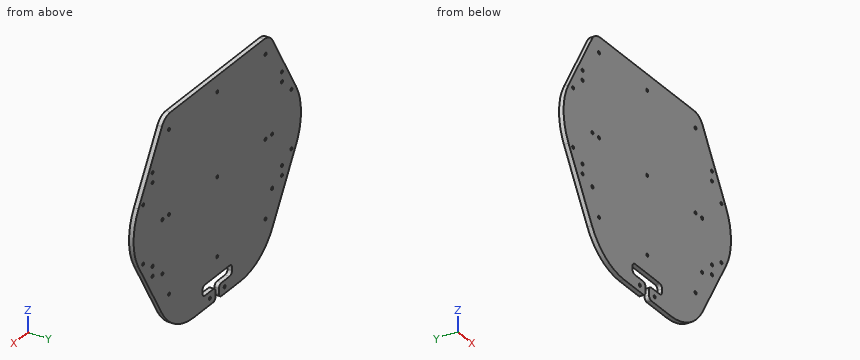
from build123d import *

# Parameters (mm, degrees)
ESBO_O1_R                = 2
ESBO_O1_R_2              = 2.1
RESSALTO_EXTRUS_O1_DEPTH = 6


with BuildPart() as part:
    # Esboço1 → Ressalto-extrusão1 (new body)
    with BuildSketch(Plane(origin=(0, 6, 0), x_dir=(1, 0, 0), z_dir=(0, 1, 0))):
        with BuildLine():
            Line((-94.999273038, -130), (94.999273038, -130))
            ThreePointArc((94.999273038, -130), (104.95780768, -127.344382024), (112.27173596, -120.082758778))
            ThreePointArc((112.27173596, -120.082758778), (112.362006236, -119.927693826), (112.451905284, -119.77241336))
            Line((112.451905284, -119.77241336), (159.951905284, -37.5))
            ThreePointArc((159.951905284, -37.5), (170, 0), (159.951905284, 37.5))
            Line((159.951905284, 37.5), (112.451905284, 119.77241336))
            ThreePointArc((112.451905284, 119.77241336), (85, 147.224318643), (47.5, 157.27241336))
            Line((47.5, 157.27241336), (8.5, 157.27241336))
            ThreePointArc((8.5, 157.27241336), (4.964466094, 155.807947265), (3.5, 152.27241336))
            Line((3.5, 152.27241336), (3.5, 145.27241336))
            ThreePointArc((3.5, 145.27241336), (4.964466094, 141.736879454), (8.5, 140.27241336))
            Line((8.5, 140.27241336), (25, 140.27241336))
            ThreePointArc((25, 140.27241336), (28.535533906, 138.807947265), (30, 135.27241336))
            Line((30, 135.27241336), (30, 131.27241336))
            ThreePointArc((30, 131.27241336), (28.535533906, 127.736879454), (25, 126.27241336))
            Line((25, 126.27241336), (-25, 126.27241336))
            ThreePointArc((-25, 126.27241336), (-28.535533906, 127.736879454), (-30, 131.27241336))
            Line((-30, 131.27241336), (-30, 135.27241336))
            ThreePointArc((-30, 135.27241336), (-28.535533906, 138.807947265), (-25, 140.27241336))
            Line((-25, 140.27241336), (-8.5, 140.27241336))
            ThreePointArc((-8.5, 140.27241336), (-4.964466094, 141.736879454), (-3.5, 145.27241336))
            Line((-3.5, 145.27241336), (-3.5, 152.27241336))
            ThreePointArc((-3.5, 152.27241336), (-4.964466094, 155.807947265), (-8.5, 157.27241336))
            Line((-8.5, 157.27241336), (-47.5, 157.27241336))
            ThreePointArc((-47.5, 157.27241336), (-85, 147.224318643), (-112.451905284, 119.77241336))
            Line((-112.451905284, 119.77241336), (-159.951905284, 37.5))
            ThreePointArc((-159.951905284, 37.5), (-170, 0), (-159.951905284, -37.5))
            Line((-159.951905284, -37.5), (-112.451905284, -119.77241336))
            ThreePointArc((-112.451905284, -119.77241336), (-112.362006236, -119.927693826), (-112.27173596, -120.082758778))
            ThreePointArc((-112.27173596, -120.082758778), (-104.95780768, -127.344382024), (-94.999273038, -130))
        make_face()
        with Locations(Location((150.5, -38.1, 0), (0, 0, 90))):
            Circle(ESBO_O1_R, mode=Mode.SUBTRACT)
        with Locations(Location((150.5, 38.1, 0), (0, 0, 90))):
            Circle(ESBO_O1_R, mode=Mode.SUBTRACT)
        with Locations(Location((-150.5, -38.1, 0), (0, 0, 90))):
            Circle(ESBO_O1_R, mode=Mode.SUBTRACT)
        with Locations(Location((-150.5, 38.1, 0), (0, 0, 90))):
            Circle(ESBO_O1_R, mode=Mode.SUBTRACT)
        with Locations(Location((15, 148.77, 0), (0, 0, 90))):
            Circle(ESBO_O1_R, mode=Mode.SUBTRACT)
        with Locations(Location((-15, 148.77, 0), (0, 0, 90))):
            Circle(ESBO_O1_R, mode=Mode.SUBTRACT)
        with Locations(Location((131.4, -57.5, 0), (0, 0, 90))):
            Circle(ESBO_O1_R, mode=Mode.SUBTRACT)
        with Locations(Location((-131.4, -57.5, 0), (0, 0, 90))):
            Circle(ESBO_O1_R, mode=Mode.SUBTRACT)
        with Locations(Location((131.4, 63, 0), (0, 0, 90))):
            Circle(ESBO_O1_R, mode=Mode.SUBTRACT)
        with Locations(Location((-131.4, 63, 0), (0, 0, 90))):
            Circle(ESBO_O1_R, mode=Mode.SUBTRACT)
        with Locations(Location((131.4, -70.2, 0), (0, 0, 90))):
            Circle(ESBO_O1_R, mode=Mode.SUBTRACT)
        with Locations(Location((-131.4, -70.2, 0), (0, 0, 90))):
            Circle(ESBO_O1_R, mode=Mode.SUBTRACT)
        with Locations(Location((131.4, 50.3, 0), (0, 0, 90))):
            Circle(ESBO_O1_R, mode=Mode.SUBTRACT)
        with Locations(Location((-131.4, 50.3, 0), (0, 0, 90))):
            Circle(ESBO_O1_R, mode=Mode.SUBTRACT)
        with Locations(Location((98, -109.22, 0), (0, 0, 90))):
            Circle(ESBO_O1_R, mode=Mode.SUBTRACT)
        with Locations(Location((111.4552, 0, 0), (0, 0, 90))):
            Circle(ESBO_O1_R_2, mode=Mode.SUBTRACT)
        with Locations(Location((111.4552, 69.85, 0), (0, 0, 90))):
            Circle(ESBO_O1_R_2, mode=Mode.SUBTRACT)
        with Locations(Location((-111.4552, 0, 0), (0, 0, 90))):
            Circle(ESBO_O1_R_2, mode=Mode.SUBTRACT)
        with Locations(Location((-111.4552, 69.85, 0), (0, 0, 90))):
            Circle(ESBO_O1_R_2, mode=Mode.SUBTRACT)
        with Locations(Location((-97.9932, 0, 0), (0, 0, 90))):
            Circle(ESBO_O1_R, mode=Mode.SUBTRACT)
        with Locations(Location((97.9932, 0, 0), (0, 0, 90))):
            Circle(ESBO_O1_R, mode=Mode.SUBTRACT)
        with Locations(Location((0, 0, 0), (0, 0, 90))):
            Circle(ESBO_O1_R, mode=Mode.SUBTRACT)
        with Locations(Location((0, -109.22, 0), (0, 0, 90))):
            Circle(ESBO_O1_R, mode=Mode.SUBTRACT)
        with Locations(Location((0, 102.4382, 0), (0, 0, 90))):
            Circle(ESBO_O1_R, mode=Mode.SUBTRACT)
        with Locations(Location((-98, 102.4382, 0), (0, 0, 90))):
            Circle(ESBO_O1_R, mode=Mode.SUBTRACT)
        with Locations(Location((98, 102.4382, 0), (0, 0, 90))):
            Circle(ESBO_O1_R, mode=Mode.SUBTRACT)
        with Locations(Location((-98, -109.22, 0), (0, 0, 90))):
            Circle(ESBO_O1_R, mode=Mode.SUBTRACT)
    extrude(amount=-RESSALTO_EXTRUS_O1_DEPTH)


solid = part.part
Design review of the part built by this model. Coordinates are the model's own, in mm. Coordinates: 2 decimals unless noted, no trailing zeros. Loops run counter-clockwise (first coordinate to the right, second up) from the corner with the lowest first, then second, coordinate; pieces in that order, holes last. Notation, with made-up numbers: (49, 44) -> (61, 44) arc R25 ccw to (61, 58) -> close; hole circle Ø3 at (87, 32). An arc over 180 degrees is marked (long way). Use a Markdown table: item, result. Add a question column.
Item 1: We need section A-A, the plane z = 96.5. Write out the cut boundary in (x, y), and give its area (3 significant figures).
Item 2: Clearance check with flat-ended pins moving along their axes: P1, Ø2, axis at y = 3, z = -51, coming from the +X side (3 decimals); P2, Ø2, axis at y = 2.5, z = 28, coming from the -X side; P3, Ø2, axis at y = 1, z = -107.5, coming from the -X side. State where each tip first meets the part, or that it passes through.
Item 3: We need section B-B, the plane y = 4.6. Count the separate pieces of the cut face and the enclosed holes in it, and give its area (3 significant figures).
Item 4: Wall thickness on L1, parallel to Z at x = 20.5, y = 1.15; L2, parallel to X at y = 4.3, z = 109.22; L3, parallel to Z at x = 150.5, y = 3.9: over which ranges is each line inside the solid? List them lowest first. Write a range as from..to.
Numbers:
| question | item | result |
|---|---|---|
| 1 | outline | (-125.89, 0) -> (125.89, 0) -> (125.89, 6) -> (-125.89, 6) -> close |
| 1 | area | 1,510 mm^2 |
| 2 | P1 | stops at x = 152.735 |
| 2 | P2 | stops at x = -164.97 |
| 2 | P3 | stops at x = -120.11 |
| 3 | separate pieces | 1 |
| 3 | enclosed holes | 27 |
| 3 | area | 77,700 mm^2 |
| 4 | L1 | z = -157.27..-140.27, -126.27..130 |
| 4 | L2 | x = -118.54..-100, -96..-2, 2..96, 100..118.54 |
| 4 | L3 | z = -53.87..-40.1, -36.1..36.1, 40.1..53.87 |
